```python
from build123d import *

# Parameters (mm, degrees)
SKETCH1_W           = 40.7
SKETCH1_H           = 20
BOSS_EXTRUDE1_DEPTH = 36.02
SKETCH3_R           = 1
BOSS_EXTRUDE2_DEPTH = 5.38
SKETCH4_W           = 3
SKETCH4_H           = 20
BOSS_EXTRUDE3_DEPTH = 7
SKETCH6_W           = 3
SKETCH6_H           = 20
BOSS_EXTRUDE4_DEPTH = 7
SKETCH7_R           = 2.7
CUT_EXTRUDE1_DEPTH  = 3


with BuildPart() as part:
    # Sketch1 → Boss-Extrude1 (new body)
    with BuildSketch(Plane.XY):
        with Locations((20.35, 10)):
            Rectangle(SKETCH1_W, SKETCH1_H)
    extrude(amount=BOSS_EXTRUDE1_DEPTH)

    # Sketch3 → Boss-Extrude2 (add)
    with BuildSketch(Plane.XY.offset(36.02)):
        with Locations(Location((30.34, 10, 0), (0, 0, 180))):
            Circle(SKETCH3_R)
    extrude(amount=BOSS_EXTRUDE2_DEPTH)

    # Sketch4 → Boss-Extrude3 (add)
    with BuildSketch(Plane(origin=(40.7, 0, 0), x_dir=(0, 0, -1), z_dir=(1, 0, 0))):
        with Locations((-29.92, 10)):
            Rectangle(SKETCH4_W, SKETCH4_H)
    extrude(amount=BOSS_EXTRUDE3_DEPTH)

    # Sketch6 → Boss-Extrude4 (add)
    with BuildSketch(Plane.ZY):
        with Locations((29.92, 10)):
            Rectangle(SKETCH6_W, SKETCH6_H)
    extrude(amount=BOSS_EXTRUDE4_DEPTH)

    # Sketch7 → Cut-Extrude1 (cut)
    with BuildSketch(Plane.XY.offset(31.42)):
        with Locations((-4.28, 14.95)):
            Circle(SKETCH7_R)
        with Locations((-4.28, 5.05)):
            Circle(SKETCH7_R)
        with Locations((44.98, 14.95)):
            Circle(SKETCH7_R)
        with Locations((44.98, 5.05)):
            Circle(SKETCH7_R)
    extrude(amount=-CUT_EXTRUDE1_DEPTH, mode=Mode.SUBTRACT)


solid = part.part
```
Geometry check sheet. Reference: the model listing, model coordinates, mm. A direction names the side the tool comes from. Give positions to 0.01 mm unless a question says otherwise; leave off trailing zeros. Write each loop counter-clockwise with the first axis right and the second up, starting at its lowest first coordinate (ties: lowest second). Pieces come first, ordered by that corner, then holes.
1) Gauge pin test, flat ends, axial feed: pin 1 (5.5 mm diameter, centred on x = -4.5, y = 12.5, fed in from +Z); pin 2 (5 mm diameter, centred on y = 4.5, z = 18.5, fed in from -X); pin 3 (4 mm diameter, centred on y = 5.5, z = 19, fed in from +X). Record the tip position at first contact, or that the pin passes through.
2) Material ranges on L1, parallel to Y at x = -4.28, z = 29.2; L2, parallel to Y at x = 44, z = 30; L3, parallel to X at y = 16, z = 27.5, recorded low to high.
3) Access from +Z, -Z, +X, -X, +Y, -Y to the whole of each face (thin tool, end or side, straight path). Record for faces 5 (the flat face through (-3, 10, 28.42)), 6 (the flat face through (-3, 10, 31.42)), 7 (the flat face through (20, 10, 0)), 8 (the flat face through (44, 10, 31.42)).
4) Section check A-A, the plane y = 5.05. State how many separate pieces and enclosed holes the cut face has, and give its area (3 significant figures).
5) Release check for a two-part mould opening along X. For faces 1 (the flat face through (40.7, 10, 14)), 2 (the cylindrical face through (47.474, 13.916, 29.941)), 3 (the flat face through (44, 10, 28.42)), 4 (the flat face through (-7, 10, 30)) record: pulls with the +X half, pulls with the -X half, needs draft (parallel to the pull), parting line crosses it, or undercut.
6) Section check D-D, the plane x = 40. Record the boundary of the cut face in (y, z), and give its area (3 significant figures).
7) Section check B-B, the plane x = -4.28. Record the boundary of the cut face in (y, z).
8) Section check C-C, the plane y = 10. Record the boundary of the cut face in (x, z), and give its area (3 significant figures).
Computed:
1. pin 1: stops at z = 31.42
1. pin 2: stops at x = 0
1. pin 3: stops at x = 40.7
2. L1: y = 0 to 2.35, 7.75 to 12.25, 17.65 to 20
2. L2: y = 0 to 2.53, 7.57 to 12.43, 17.47 to 20
2. L3: x = 0 to 40.7
3. face 5: -Z, -X, +Y, -Y
3. face 6: +Z, -X, +Y, -Y
3. face 7: -Z, +X, -X, +Y, -Y
3. face 8: +Z, +X, +Y, -Y
4. separate pieces: 3
4. enclosed holes: 0
4. area: 1,480 mm2
5. face 1: pulls with the +X half
5. face 2: undercut
5. face 3: needs draft
5. face 4: pulls with the -X half
6. outline: (0, 0) - (20, 0) - (20, 36.02) - (0, 36.02) - close
6. area: 720 mm2
7. outline: (0, 28.42) - (2.35, 28.42) - (2.35, 31.42) - (0, 31.42) - close; (7.75, 28.42) - (12.25, 28.42) - (12.25, 31.42) - (7.75, 31.42) - close; (17.65, 28.42) - (20, 28.42) - (20, 31.42) - (17.65, 31.42) - close
8. outline: (-7, 28.42) - (0, 28.42) - (0, 0) - (40.7, 0) - (40.7, 28.42) - (47.7, 28.42) - (47.7, 31.42) - (40.7, 31.42) - (40.7, 36.02) - (31.34, 36.02) - (31.34, 41.4) - (29.34, 41.4) - (29.34, 36.02) - (0, 36.02) - (0, 31.42) - (-7, 31.42) - close
8. area: 1,520 mm2
